Source: CAD feature listing. Evaluate the final solid. Frame: model axes, mm. A direction names the side the tool comes from. Coordinates: 2 decimals unless noted, no trailing zeros. Loops run counter-clockwise (first coordinate to the right, second up) from the corner with the lowest first, then second, coordinate; pieces in that order, holes last. Notation, with made-up numbers: (33.25, 59.5) - (48.25, 59.5) arc R24 cw to (48.25, 91.5) - close; hole circle Ø11 at (-20, 18). An arc over 180 degrees is marked (long way). Use CSV: the item, a comma, the result in double quotes. Start each with the question number.
```python
from build123d import *

# Parameters (mm, degrees)
SKETCH1_R           = 0.4
BOSS_EXTRUDE1_DEPTH = 9
SKETCH2_R           = 9.25
BOSS_EXTRUDE2_DEPTH = 3


with BuildPart() as part:
    # Sketch1 → Boss-Extrude1 (new body)
    with BuildSketch(Plane(origin=(0, 0, 0), x_dir=(1, 0, 0), z_dir=(0, 1, 0))):
        with BuildLine():
            add(Edge.make_bspline(
                [(-5.065227978, 4.461610195), (-5.526615005, 4.86619147), (-5.830003112, 5.39406146), (-5.975392301, 6.045220165)],
                knots=[0, 0, 0, 0, 0.872429449, 0.872429449, 0.872429449, 0.872429449], degree=3))
            ThreePointArc((-5.065227978, 4.461610195), (-5.560258819, 3.827012132), (-5.976238464, 3.138004752))
            add(Edge.make_bspline(
                [(-7.780961116, 3.42149735), (-7.125870497, 3.507536778), (-6.52429628, 3.413039245), (-5.976238464, 3.138004752)],
                knots=[0.127683247, 0.127683247, 0.127683247, 0.127683247, 1, 1, 1, 1], degree=3))
            ThreePointArc((-7.780961116, 3.42149735), (-7.951879756, 3.00293329), (-8.10030101, 2.575873357))
            add(Edge.make_bspline(
                [(-6.558450277, 1.596630818), (-7.155006493, 1.740452504), (-7.668956737, 2.066866683), (-8.10030101, 2.575873357)],
                knots=[0, 0, 0, 0, 0.872429449, 0.872429449, 0.872429449, 0.872429449], degree=3))
            ThreePointArc((-6.558450277, 1.596630818), (-6.701865893, 0.804669837), (-6.749999881, 0.00126872))
            add(Edge.make_bspline(
                [(-8.479748007, -0.586407486), (-7.939678588, -0.205787566), (-7.363095879, -0.009895497), (-6.749999881, 0.00126872)],
                knots=[0.127683247, 0.127683247, 0.127683247, 0.127683247, 1, 1, 1, 1], degree=3))
            ThreePointArc((-8.479748007, -0.586407486), (-8.436572529, -1.036457408), (-8.369528376, -1.483574994))
            add(Edge.make_bspline(
                [(-6.549210655, -1.634117437), (-7.144272221, -1.784003157), (-7.751044795, -1.733822342), (-8.369528376, -1.483574994)],
                knots=[0, 0, 0, 0, 0.872429449, 0.872429449, 0.872429449, 0.872429449], degree=3))
            ThreePointArc((-6.549210655, -1.634117437), (-6.308156258, -2.402012621), (-5.977417671, -3.13575796))
            add(Edge.make_bspline(
                [(-7.235926822, -4.459973434), (-6.934601997, -3.871968458), (-6.515098947, -3.4305633), (-5.977417671, -3.13575796)],
                knots=[0.127683247, 0.127683247, 0.127683247, 0.127683247, 1, 1, 1, 1], degree=3))
            ThreePointArc((-7.235926822, -4.459973434), (-6.988548208, -4.838408204), (-6.721397655, -5.203154193))
            add(Edge.make_bspline(
                [(-5.039625799, -4.490509081), (-5.496871281, -4.899765193), (-6.0574619, -5.137313564), (-6.721397655, -5.203154193)],
                knots=[0, 0, 0, 0, 0.872429449, 0.872429449, 0.872429449, 0.872429449], degree=3))
            ThreePointArc((-5.039625799, -4.490509081), (-4.469324045, -5.058422935), (-3.835481109, -5.554420281))
            add(Edge.make_bspline(
                [(-4.334442004, -7.311813216), (-4.34089166, -6.651128039), (-4.174571361, -6.065330394), (-3.835481109, -5.554420281)],
                knots=[0.127683247, 0.127683247, 0.127683247, 0.127683247, 1, 1, 1, 1], degree=3))
            ThreePointArc((-4.334442004, -7.311813216), (-3.939531713, -7.53193799), (-3.533475733, -7.730753472))
            add(Edge.make_bspline(
                [(-2.375523406, -6.318179211), (-2.590203375, -6.893050073), (-2.976187484, -7.36390816), (-3.533475733, -7.730753472)],
                knots=[0, 0, 0, 0, 0.872429449, 0.872429449, 0.872429449, 0.872429449], degree=3))
            ThreePointArc((-2.375523406, -6.318179211), (-1.606623554, -6.556009515), (-0.814882047, -6.700631854))
            add(Edge.make_bspline(
                [(-0.439988759, -8.488604708), (-0.752735357, -7.906594341), (-0.877699786, -7.31060339), (-0.814882047, -6.700631854)],
                knots=[0.127683247, 0.127683247, 0.127683247, 0.127683247, 1, 1, 1, 1], degree=3))
            ThreePointArc((-0.439988759, -8.488604708), (0.011984021, -8.499991552), (0.463922896, -8.487330296))
            add(Edge.make_bspline(
                [(0.832782771, -6.698430626), (0.909848909, -7.307220251), (0.786895617, -7.903520141), (0.463922896, -8.487330296)],
                knots=[0, 0, 0, 0, 0.872429449, 0.872429449, 0.872429449, 0.872429449], degree=3))
            ThreePointArc((0.832782771, -6.698430626), (1.624135031, -6.551693323), (2.392396671, -6.311809421))
            add(Edge.make_bspline(
                [(3.555260608, -7.72075916), (3.007863545, -7.350755165), (2.620242233, -6.881105252), (2.392396671, -6.311809421)],
                knots=[0.127683247, 0.127683247, 0.127683247, 0.127683247, 1, 1, 1, 1], degree=3))
            ThreePointArc((3.555260608, -7.72075916), (3.96075436, -7.520799485), (4.355042381, -7.299562032))
            add(Edge.make_bspline(
                [(3.850308451, -5.54415231), (4.201465773, -6.047394331), (4.369710416, -6.632530905), (4.355042381, -7.299562032)],
                knots=[0, 0, 0, 0, 0.872429449, 0.872429449, 0.872429449, 0.872429449], degree=3))
            ThreePointArc((3.850308451, -5.54415231), (4.482823853, -5.046463148), (5.051606144, -4.477027515))
            add(Edge.make_bspline(
                [(6.736042616, -5.184180734), (6.079397157, -5.110946566), (5.517918333, -4.875228826), (5.051606144, -4.477027515)],
                knots=[0.127683247, 0.127683247, 0.127683247, 0.127683247, 1, 1, 1, 1], degree=3))
            ThreePointArc((6.736042616, -5.184180734), (7.002163607, -4.818682892), (7.24847414, -4.439552076))
            add(Edge.make_bspline(
                [(5.985774866, -3.119775513), (6.530577461, -3.402183249), (6.951477219, -3.84210877), (7.24847414, -4.439552076)],
                knots=[0, 0, 0, 0, 0.872429449, 0.872429449, 0.872429449, 0.872429449], degree=3))
            ThreePointArc((5.985774866, -3.119775513), (6.314551754, -2.385149082), (6.553553527, -1.616612559))
            add(Edge.make_bspline(
                [(8.373678438, -1.459968977), (7.758214146, -1.700281702), (7.151505842, -1.75249623), (6.553553527, -1.616612559)],
                knots=[0.127683247, 0.127683247, 0.127683247, 0.127683247, 1, 1, 1, 1], degree=3))
            ThreePointArc((8.373678438, -1.459968977), (8.439461558, -1.01266412), (8.481367828, -0.562494242))
            add(Edge.make_bspline(
                [(6.749972396, 0.019304256), (7.363612555, 0.022427015), (7.940744366, -0.171505818), (8.481367828, -0.562494242)],
                knots=[0, 0, 0, 0, 0.872429449, 0.872429449, 0.872429449, 0.872429449], degree=3))
            ThreePointArc((6.749972396, 0.019304256), (6.699691947, 0.822573894), (6.554160776, 1.614148852))
            add(Edge.make_bspline(
                [(8.093005444, 2.598704077), (7.65971777, 2.099897208), (7.146769547, 1.771712133), (6.554160776, 1.614148852)],
                knots=[0.127683247, 0.127683247, 0.127683247, 0.127683247, 1, 1, 1, 1], degree=3))
            ThreePointArc((8.093005444, 2.598704077), (7.943380571, 3.025343799), (7.771282357, 3.443424244))
            add(Edge.make_bspline(
                [(5.967832596, 3.153961653), (6.509732754, 3.44189952), (7.110882674, 3.53838705), (7.771282357, 3.443424244)],
                knots=[0, 0, 0, 0, 0.872429449, 0.872429449, 0.872429449, 0.872429449], degree=3))
            ThreePointArc((5.967832596, 3.153961653), (5.550013455, 3.841855105), (5.053288778, 4.475128213))
            add(Edge.make_bspline(
                [(5.958322434, 6.062045345), (5.806472362, 5.419014975), (5.504794477, 4.890042598), (5.053288778, 4.475128213)],
                knots=[0.127683247, 0.127683247, 0.127683247, 0.127683247, 1, 1, 1, 1], degree=3))
            ThreePointArc((5.958322434, 6.062045345), (5.627566824, 6.370281912), (5.280889753, 6.660495734))
            add(Edge.make_bspline(
                [(3.818534268, 5.566084444), (4.16455163, 6.072874324), (4.652003458, 6.437678087), (5.280889753, 6.660495734)],
                knots=[0, 0, 0, 0, 0.872429449, 0.872429449, 0.872429449, 0.872429449], degree=3))
            ThreePointArc((3.818534268, 5.566084444), (3.128893766, 5.98101361), (2.394769219, 6.310909632))
            add(Edge.make_bspline(
                [(2.45865956, 8.136645081), (2.623034112, 7.496701718), (2.601737332, 6.888123235), (2.394769219, 6.310909632)],
                knots=[0.127683247, 0.127683247, 0.127683247, 0.127683247, 1, 1, 1, 1], degree=3))
            ThreePointArc((2.45865956, 8.136645081), (2.022545337, 8.25586521), (1.580708948, 8.351727918))
            add(Edge.make_bspline(
                [(0.794455758, 6.703084368), (0.865321915, 7.312626807), (1.127406312, 7.862174657), (1.580708948, 8.351727918)],
                knots=[0, 0, 0, 0, 0.872429449, 0.872429449, 0.872429449, 0.872429449], degree=3))
            ThreePointArc((0.794455758, 6.703084368), (-0.009017778, 6.749993976), (-0.812363108, 6.700937709))
            add(Edge.make_bspline(
                [(-1.604252589, 8.347237485), (-1.161309642, 7.856984441), (-0.897346481, 7.308217849), (-0.812363108, 6.700937709)],
                knots=[0.127683247, 0.127683247, 0.127683247, 0.127683247, 1, 1, 1, 1], degree=3))
            ThreePointArc((-1.604252589, 8.347237485), (-2.045816912, 8.250129282), (-2.481593228, 8.129679886))
            add(Edge.make_bspline(
                [(-2.411622992, 6.304488444), (-2.632142622, 6.877144615), (-2.655466033, 7.485541762), (-2.481593228, 8.129679886)],
                knots=[0, 0, 0, 0, 0.872429449, 0.872429449, 0.872429449, 0.872429449], degree=3))
            ThreePointArc((-2.411622992, 6.304488444), (-3.144863458, 5.972632069), (-3.833392837, 5.555861712))
            add(Edge.make_bspline(
                [(-5.299649804, 6.645578377), (-4.679611352, 6.417326717), (-4.19085903, 6.054087828), (-3.833392837, 5.555861712)],
                knots=[0.127683247, 0.127683247, 0.127683247, 0.127683247, 1, 1, 1, 1], degree=3))
            ThreePointArc((-5.299649804, 6.645578377), (-5.645507162, 6.35438816), (-5.975392301, 6.045220165))
        make_face()
        Circle(SKETCH1_R, mode=Mode.SUBTRACT)
    extrude(amount=BOSS_EXTRUDE1_DEPTH)

    # Sketch2 → Boss-Extrude2 (add)
    with BuildSketch(Plane.XZ):
        Circle(SKETCH2_R)
    extrude(amount=BOSS_EXTRUDE2_DEPTH)


solid = part.part
```
(1) Section C-C on y = -2. Output: boundary loops of the cut face in (x, z), plus the area to 3 significant figures.
(2) Section B-B on z = -1. Output: boundary loops of the cut face in (x, y).
(3) Draft query along X for faces 6 (the cylindrical face through (6.7, 4.44, -0.81)), 7 (the cylindrical face through (0, 4.44, -6.75)), 8 (the cylindrical face through (-2.04, 4.44, -8.25)). Return one class per face: released by +X, released by -X, zero draft, split by the parting line, or undercut.
(4) Reachability of faces 1 (the cylindrical face through (7.946, 4.437, -3.019)), 2 (the cylindrical face through (-7.95, 4.44, -3.01)), 3 (the cylindrical face through (-3.945, 4.437, 7.529)), 4 (the cylindrical face through (8.44, 4.44, 1.02)), 5 (the cylindrical face through (5.56, 4.44, -3.83)) from +Z, -Z, +X, -X, +Y, -Y: full face, straight path, thin tool, end or side. Return the list, or none.
(5) Section A-A on x = 0. Output: boundary loops of the cut face in (y, z).
(6) Pin query (flat end, axial travel): pin 1 Ø5 at (y, z) = (3.5, -7) entering from +X; pin 2 Ø1.5 at (y, z) = (-1, -2) entering from -X. Return the tip coordinate at first contact, or that it passes through.
(7) Ray query, line 1 (Z direction, x = 0, y = 3.25); line 2 (Y direction, x = -5.25, z = 7.5); line 3 (X direction, y = 2.5, z = -7.75). Return the intervals inside material, ascending. Write a range as [from, to].
Solution:
1,outline,"circle Ø18.5 at (0, 0)"
1,area,"269 mm²"
2,outline,"(-9.2, -3) - (9.2, -3) - (9.2, 0) - (6.68, 0) - (6.68, 9) - (-6.68, 9) - (-6.68, 0) - (-9.2, 0) - close"
3,face 6,"released by +X"
3,face 7,"undercut"
3,face 8,"released by -X"
4,face 1,"-Z, +X, +Y"
4,face 2,"-Z, -X, +Y"
4,face 3,"+Z, -X, +Y"
4,face 4,"+Z, +X, +Y"
4,face 5,"+Y"
5,outline,"(-3, -9.25) - (0, -9.25) - (0, -6.75) - (9, -6.75) - (9, -0.4) - (0, -0.4) - (0, 0.4) - (9, 0.4) - (9, 8.5) - (0, 8.5) - (0, 9.25) - (-3, 9.25) - close"
6,pin 1,"stops at x = 5.96"
6,pin 2,"stops at x = -9.17"
7,line 1,"z = [-6.75, -0.4], [0.4, 8.5]"
7,line 2,"y = [-3, 0]"
7,line 3,"x = [-2.56, -1.17], [1.14, 2.54]"
